from build123d import *

# Parameters (mm, degrees)
SKETCH1_R           = 10.75
BOSS_EXTRUDE1_DEPTH = 73.5
SKETCH2_R           = 3
BOSS_EXTRUDE2_DEPTH = 1
CUT_EXTRUDE1_START  = -0.05
SKETCH2_3_R         = 7
SKETCH2_3_R_2       = 3
CUT_EXTRUDE1_DEPTH  = 0.05
SKETCH3_R           = 7.5
CUT_EXTRUDE2_DEPTH  = 0.05
FILLET1_R           = 2
FILLET2_R           = 1


with BuildPart() as part:
    # Sketch1 → Boss-Extrude1 (new body)
    with BuildSketch(Plane.XY):
        Circle(SKETCH1_R)
    extrude(amount=BOSS_EXTRUDE1_DEPTH)

    # Sketch2 → Boss-Extrude2 (add)
    with BuildSketch(Plane.XY.offset(73.5)):
        Circle(SKETCH2_R)
    extrude(amount=BOSS_EXTRUDE2_DEPTH)

    # Sketch2<3> → Cut-Extrude1 (cut)
    with BuildSketch(Plane.XY.offset(73.5).offset(CUT_EXTRUDE1_START)):
        Circle(SKETCH2_3_R)
        Circle(SKETCH2_3_R_2, mode=Mode.SUBTRACT)
    extrude(amount=CUT_EXTRUDE1_DEPTH, mode=Mode.SUBTRACT)

    # Sketch3 → Cut-Extrude2 (cut)
    with BuildSketch(Plane(origin=(0, 0, 0), x_dir=(-1, 0, 0), z_dir=(0, 0, -1))):
        Circle(SKETCH3_R)
    extrude(amount=-CUT_EXTRUDE2_DEPTH, mode=Mode.SUBTRACT)

    # Fillet1
    fillet1_edges = [part.edges().sort_by_distance(p)[0] for p in [
        (-10.75, 0, 0),
        (-10.75, 0, 73.5),
    ]]
    fillet(fillet1_edges, radius=FILLET1_R)

    # Fillet2
    fillet2_edges = [part.edges().sort_by_distance(p)[0] for p in [
        (-3, 0, 74.5),
    ]]
    fillet(fillet2_edges, radius=FILLET2_R)


solid = part.part
Input: part model. Units: mm. Frame: model coordinates. A direction names the side the tool comes from. Give positions to 0.01 mm unless a question says otherwise; leave off trailing zeros. Loops run counter-clockwise (first coordinate to the right, second up) from the corner with the lowest first, then second, coordinate; pieces in that order, holes last. Notation, with made-up numbers: (9.5, 38) -> (49.5, 38) arc R10 cw to (49.5, 53) -> close; hole circle Ø10 at (47, -38). An arc over 180 degrees is marked (long way). Answer as a JSON object with one key per item and string values. Group by question number.
Item 1: Pull-direction query (Y, two-part tool) for faces 1 (the flat face through (0, 0, 74.5)), 2 (the cylindrical face through (-1.4, 10.66, 36.26)), 3 (the flat face through (0, 0, 0.05)); classes: released by +Y, released by -Y, zero draft, split by the parting line, or undercut.
Item 2: Cut plane A-A, the plane z = 8.5. Return the cut outline in (x, y), and give its area (3 significant figures).
Item 3: Reachability of faces 4 (the flat face through (1, -3, 73.45)), 5 (the flat face through (-4, 7, 0)) from +Z, -Z, +X, -X, +Y, -Y: full face, straight path, thin tool, end or side. Return the list, or none.
Item 4: Line query: probe 1 along Z at (x, y) = (-5.5, -2.75); probe 2 along Z at (x, y) = (9.25, 0); probe 3 along Y at (x, z) = (0, 73.55). Output: solid intervals per line, ascending.
Item 5: Pin query (flat end, axial travel): P1, Ø8.5, axis at x = 0, y = 0, coming from the -Z side; P2, Ø12, axis at x = -8.5, z = 37.5, coming from the +Y side; P3, Ø8, axis at x = -7, z = 47, coming from the +Y side. Return the tip coordinate at first contact, or that it passes through.
Checks:
{
 "1": {"face 1": "zero draft", "face 2": "split by the parting line", "face 3": "undercut"},
 "2": {"outline": "circle Ø21.5 at (0, 0)", "area": "363 mm²"},
 "3": {"face 4": "+Z", "face 5": "-Z, +X, -X, +Y, -Y"},
 "4": {"probe 1": "z = 0.05 to 73.45", "probe 2": "z = 0.06 to 73.44", "probe 3": "y = -3 to 3"},
 "5": {"P1": "stops at z = 0.05", "P2": "stops at y = 10.46", "P3": "stops at y = 10.32"}
}
